Work out the finished part from the listing and answer in its coordinate system (mm). Face numbers are marked on the shaded views. Give positions to 0.01 mm unless a question says otherwise; leave off trailing zeros. Loops run counter-clockwise (first coordinate to the right, second up) from the corner with the lowest first, then second, coordinate; pieces in that order, holes last.
from build123d import *

# Parameters (mm, degrees)
SKETCH1_W          = 9.525
SKETCH1_H          = 2.0828
CHAMFER1_SIZE      = 0.5953125
CUT_EXTRUDE2_DEPTH = 1.54686


with BuildPart() as part:
    # Sketch1 → Revolve1 (revolve)
    with BuildSketch(Plane(origin=(0, 0, 0), x_dir=(0, 0, -1), z_dir=(1, 0, 0))):
        with Locations((6.9723, 1.0414)):
            Rectangle(SKETCH1_W, SKETCH1_H)
    revolve(axis=Axis((0, 0, -11.7348), (0, 0, 1)))

    # Chamfer1
    chamfer1_edges = [part.edges().sort_by_distance(p)[0] for p in [
        (0, -2.0828, -11.7348),
    ]]
    chamfer(chamfer1_edges, length=CHAMFER1_SIZE)

    # Sketch7 → Revolve2 (revolve)
    with BuildSketch(Plane(origin=(0, 0, 0), x_dir=(0, 0, -1), z_dir=(1, 0, 0)), mode=Mode.PRIVATE) as revolve2_sk:
        with BuildLine():
            Line((1.87833, 3.9624), (2.2098, 3.9624))
            Line((2.2098, 3.9624), (2.2098, 0))
            Line((2.2098, 0), (0, 0))
            Line((0, 0), (0, 2.0828))
            ThreePointArc((0, 2.0828), (0.796523813, 3.165144808), (1.87833, 3.9624))
        make_face()
    revolve(revolve2_sk.sketch.rotate(Axis((0, 0, 0), (0, 0, -1)), 180), axis=Axis((0, 0, 0), (0, 0, -1)))

    # Sketch5 → Cut-Extrude2 (cut)
    with BuildSketch(Plane.XY):
        Polygon((1.190625, -0.687407664), (1.190625, 0.687407664), (0, 1.374815329), (-1.190625, 0.687407664), (-1.190625, -0.687407664), (0, -1.374815329), align=None)
    extrude(amount=-CUT_EXTRUDE2_DEPTH, mode=Mode.SUBTRACT)

    # Cut-Extrude3 cone 1 section (on through the dimple's axis) → Cut-Extrude3 (revolve, cut)
    with BuildSketch(Plane(origin=(0, 0, 0), x_dir=(0, -1, 0), z_dir=(1, 0, 0))):
        Polygon((0, 0), (1.374815329, 0), (0, 1.374815329), align=None)
    revolve(axis=Axis((0, 0, 0), (0, 0, -1)), mode=Mode.SUBTRACT)


solid = part.part
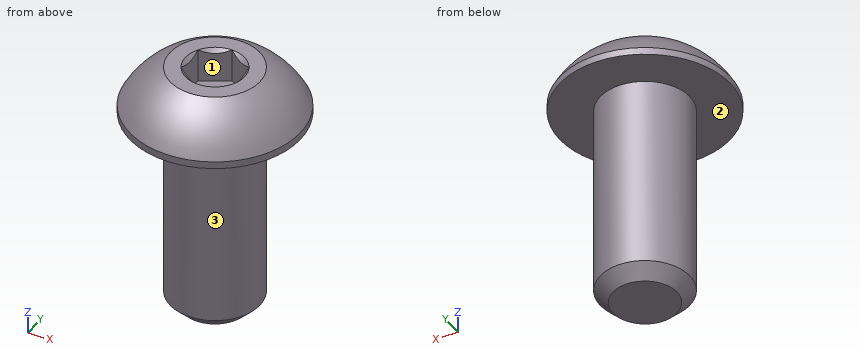
Item 1: Find section A-A, the plane y = 0. Write down the section's boundary in (x, z), plus the area to 3 significant figures.
Item 2: Find section C-C, the plane x = 2.75. Write down the section's boundary in (y, z), plus the area to 3 significant figures.
Item 3: Determine the mould class of the marked faces 1, 2 and 3 for opening direction Y: released by +Y, released by -Y, zero draft, split by the parting line, or undercut.
Item 4: Consider line 1 (Z direction, x = -1, y = -0.25); line 2 (Y direction, x = 0, z = -10.5); line 3 (Y direction, x = 2.5, z = -2). Determine where each line is inside the solid, lowest interval first.
Item 5: Flat-ended cylindrical pins translate along their axes: pin 1 Ø3 at (y, z) = (-3, -7.5) entering from -X (3 decimals); pin 2 Ø1 at (x, y) = (-0.5, 2) entering from -Z; pin 3 Ø2 at (x, z) = (-2.5, -4.5) entering from +Y (3 decimals). Find the tip coordinate at first contact, or state that the pin passes through.
Item 6: Find section B-B, the plane z = -3. Write down the section's boundary in (x, y).
Item 7: Find section D-D, the plane y = 2.5. Write down the section's boundary in (x, z), plus the area to 3 significant figures.
Ans:
1. outline: (-3.96, -2.21) - (-2.08, -2.21) - (-2.08, -11.14) - (-1.49, -11.73) - (1.49, -11.73) - (2.08, -11.14) - (2.08, -2.21) - (3.96, -2.21) - (3.96, -1.88) arc R4.48 ccw to (2.08, 0) - (1.37, 0) - (1.19, -0.18) - (1.19, -1.55) - (-1.19, -1.55) - (-1.19, -0.18) - (-1.37, 0) - (-2.08, 0) arc R4.48 ccw to (-3.96, -1.88) - close
1. area: 50.3 mm2
2. outline: (-2.85, -2.21) - (2.85, -2.21) - (2.85, -1.88) arc R3.53 ccw to (-2.85, -1.88) - close
2. area: 7.67 mm2
3. face 1: undercut
3. face 2: zero draft
3. face 3: split by the parting line
4. line 1: z = -11.73 to -1.55
4. line 2: y = -2.08 to 2.08
4. line 3: y = -3.07 to 3.07
5. pin 1: stops at x = -1.445
5. pin 2: stops at z = -11.66
5. pin 3: stops at y = 1.445
6. outline: circle Ø4.17 at (0, 0)
7. outline: (-3.07, -2.21) - (3.07, -2.21) - (3.07, -1.88) arc R3.71 ccw to (-3.07, -1.88) - close
7. area: 9.08 mm2
